from build123d import *

# Parameters (mm, degrees)
F0_W     = 762
F0_H     = 660.4
F1_DEPTH = 12.7
F2_R     = 50.8
F2_R_2   = 57.15
F3_DEPTH = 12.701
F4_R     = 187.325
F4_R_2   = 180.975
F5_DEPTH = 6.35


with BuildPart() as f1:
    # F0 (on Top) → F1 (new body)
    with BuildSketch(Plane.XY):
        with Locations((-381, 330.2)):
            Rectangle(F0_W, F0_H)
    extrude(amount=F1_DEPTH)

    # F2 (on face) → F3 (cut, through all)
    with BuildSketch(Plane.XY.offset(12.7)):
        with Locations((-139.7, 330.2)):
            Circle(F2_R)
        with Locations((-279.4, 330.2)):
            Circle(F2_R)
        with Locations((-400.05, 330.2)):
            Circle(F2_R_2)
        with Locations((-520.7, 330.2)):
            Circle(F2_R_2)
        with Locations((-654.05, 330.2)):
            Circle(F2_R_2)
    extrude(amount=-F3_DEPTH, mode=Mode.SUBTRACT)

    # F4 (on face) → F5 (cut)
    with BuildSketch(Plane.XY.offset(12.7)):
        with BuildLine():
            Line((-762, 0), (-400.050008, 0))
            ThreePointArc((-400.050008, 0), (-69.850008, 330.2), (-400.050008, 660.4))
            Line((-400.050008, 660.4), (-762, 660.4))
            Line((-762, 660.4), (-762, 0))
        make_face()
        with BuildLine():
            ThreePointArc((-400.050008, 654.050008), (-76.2, 330.2), (-400.050008, 6.349992))
            Line((-400.050008, 6.349992), (-755.65, 6.349992))
            Line((-755.65, 6.349992), (-755.65, 654.050008))
            Line((-755.65, 654.050008), (-400.050008, 654.050008))
        make_face(mode=Mode.SUBTRACT)
        with Locations((-403.225, 330.2)):
            Circle(F4_R)
        with Locations((-403.225, 330.2)):
            Circle(F4_R_2, mode=Mode.SUBTRACT)
    extrude(amount=-F5_DEPTH, mode=Mode.SUBTRACT)


solid = f1.part
CAD build for the part. Positions are in the model's coordinates, mm. A direction names the side the tool comes from. Give positions to 0.01 mm unless a question says otherwise; leave off trailing zeros. Loops run counter-clockwise (first coordinate to the right, second up) from the corner with the lowest first, then second, coordinate; pieces in that order, holes last. Notation, with made-up numbers: M 29.25,11 L 34.25,11 A22 ccw 34.25,28 Z; hole C 24.5,6.25 d4. An arc over 180 degrees is marked long. Answer in a Markdown table with one row per item. Add a question column.
Item 1: Probe probe 1 along Y at (x, z) = (-520.7, 3.5); probe 2 along Y at (x, z) = (-106.5, 9); probe 3 along Y at (x, z) = (-139.7, 6). List the from-to ranges inside material, lowest first.
Item 2: Tool access for faces 1 (the face through (-557, 428, 6.35)), 2 (the face through (-445.402, 295.425, 6.439)): list every direction of +Z, -Z, +X, -X, +Y, -Y with a clear straight run to the whole face (end or side of a thin tool).
Item 3: Band-saw the part on B-B on x = -654.05. Give the cut face in (y, z), then the cut area to 3 significant figures.
Item 4: Band-saw the part on A-A on z = 10.5. Give the number of separate pieces and of enclosed holes in the cut face, then the cut area to 3 significant figures.
Item 5: Band-saw the part on D-D on x = -279.4. Give the cut face in (y, z), then the cut area to 3 significant figures.
Item 6: Drop flat-ended pins along their axis: P1, Ø1, axis at y = 303.5, z = 7, coming from the -X side; P2, Ø3, axis at x = -494.5, z = 10, coming from the -Y side; P3, Ø1.5, axis at x = -602, z = 11, coming from the +Y side; P4, Ø1.5, axis at x = -511.5, y = 83.5, coming from the -Z side. Give the stop position or say it passes through.
Item 7: Mould opens along X. For faces 3 (the face through (-467.91, 308.31, 6.44)), 4 (the face through (-572, 191, 12.7)) say: +X half, -X half, draft (parallel to the pull), parting line (faces both ways), or undercut.
Reply:
| question | item | result |
|---|---|---|
| 1 | probe 1 | y = 0 to 273.05, 387.35 to 660.4 |
| 1 | probe 2 | y = 0 to 179, 193.43 to 291.75, 368.65 to 466.97, 481.4 to 660.4 |
| 1 | probe 3 | y = 0 to 279.4, 381 to 660.4 |
| 2 | face 1 | +Z |
| 2 | face 2 | +Z, -Z |
| 3 | outline | M 0,0 L 273.05,0 L 273.05,12.7 L 6.35,12.7 L 6.35,6.35 L 0,6.35 Z; M 387.35,0 L 660.4,0 L 660.4,6.35 L 654.05,6.35 L 654.05,12.7 L 387.35,12.7 Z |
| 3 | area | 6,850 mm^2 |
| 4 | separate pieces | 3 |
| 4 | enclosed holes | 6 |
| 4 | area | 434,000 mm^2 |
| 5 | outline | M 0,0 L 279.4,0 L 279.4,12.7 L 198.22,12.7 L 198.22,6.35 L 189.64,6.35 L 189.64,12.7 L 29.66,12.7 L 29.66,6.35 L 22.83,6.35 L 22.83,12.7 L 0,12.7 Z; M 381,0 L 660.4,0 L 660.4,12.7 L 637.57,12.7 L 637.57,6.35 L 630.74,6.35 L 630.74,12.7 L 470.76,12.7 L 470.76,6.35 L 462.18,6.35 L 462.18,12.7 L 381,12.7 Z |
| 5 | area | 6,900 mm^2 |
| 6 | P1 | stops at x = -755.65 |
| 6 | P2 | stops at y = 6.35 |
| 6 | P3 | stops at y = 654.05 |
| 6 | P4 | stops at z = 0 |
| 7 | face 3 | undercut |
| 7 | face 4 | draft |
